Autodesk Inventor part; units mm, degrees
ref_plane "YZ Plane" through (0, 0, 0) normal (1, 0, 0) x (0, 1, 0)
ref_plane "XZ Plane" through (0, 0, 0) normal (0, 1, 0) x (-1, 0, 0)
ref_plane "XY Plane" through (0, 0, 0) normal (0, 0, 1) x (1, 0, 0)
sketch "Sketch2" plane through (0, 0, 0) normal (1, 0, 0) x (0, 1, 0)
  line L0 (0, 0) -> (30, 0)
  line L1 (30, 60) -> (30, -60)
  line L2 (30, 60) -> (27, 60)
  line L3 (27, 60) -> (27, -60)
  line L4 (27, -60) -> (30, -60)
  line L5 (27, 60) -> (0, 60)
  line L6 (0, 60) -> (5, 60)
  line L7 (5, 60) -> (5, 54)
  line L8 (5, 54) -> (27, 54)
  line L9 (27, -60) -> (0, -60)
  line L10 (0, -60) -> (5, -60)
  line L11 (5, -60) -> (5, -54)
  line L12 (5, -54) -> (27, -54)
  line L13 (0, 60) -> (0, -60)
  line L14 (27, 0) -> (28, 0)
  line L15 (28, 0) -> (28, -3)
  line L16 (28, -3) -> (27, -3)
  line L17 (28, 0) -> (28, 2)
  line L18 (28, 2) -> (30, 2)
  line L19 (30, 2) -> (28, 0)
  line L20 (28, 0) -> (28, -2)
  line L21 (28, -2) -> (30, -2)
  line L22 (30, -2) -> (28, 0)
  line L23 (5, -54) -> (0, -54)
  dimension "d12" = 30
  dimension "d13" = 120
  dimension "d14" = 3
  dimension "d15" = 5
  dimension "d16" = 6
  dimension "d17" = 6
  dimension "d26" = 1
  dimension "d27" = 3
  dimension "d28" = 2
  dimension "d29" = 2
revolve "Revolution1" add sketch "Sketch2" angle 360 about axis through (0, 0, 60) along (0, 0, -1) contours L23 L11 L9 L13 | L22 L21 L15 | L16 L15 L21 L1 L4 L3 | L12 L3 L9 L11
fillet "Fillet2" radius 3 1 edges at (0, -30, -60)
fillet "Fillet3" radius 3 1 edges at (0, -27, -54)
properties part number "Plenum"
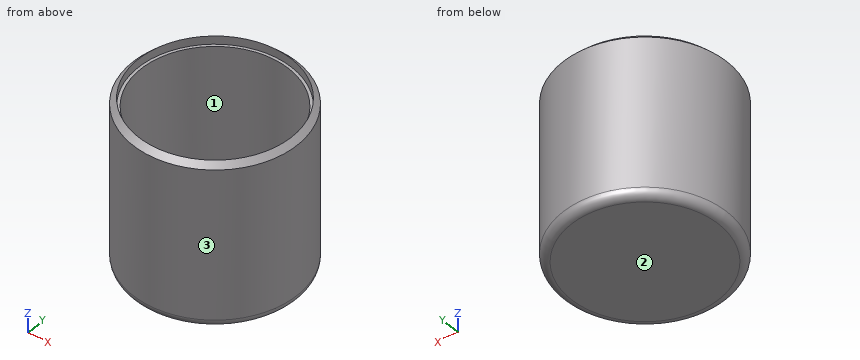
Build history of the part. All positions in model axes, mm. Face numbers are marked on the shaded views. Give positions to 0.01 mm unless a question says otherwise; leave off trailing zeros. Loops run counter-clockwise (first coordinate to the right, second up) from the corner with the lowest first, then second, coordinate; pieces in that order, holes last.
Item 1: Drill centre lines: line 1 (X direction, y = 0, z = -2); line 2 (X direction, y = 0, z = -23); line 3 (Z direction, x = 14, y = -6). Where is each one in solid material? Low to high.
Answers follow:
line 1: x = -30 to -28, 28 to 30
line 2: x = -30 to -27, 27 to 30
line 3: z = -60 to -54
Item 2: Pull direction X, two halves, no side cores. Call the marked faces 1, 2 and 3: released by +X, released by -X, zero draft, split by the parting line, or undercut.
Answers follow:
face 1: undercut
face 2: zero draft
face 3: split by the parting line
Item 3: Slice it at A-A, the plane y = 0. List the corners of the cut face in (x, z), and give its area (3 significant figures).
Answers follow:
outline: (-30, -57) arc R3 ccw to (-27, -60) - (27, -60) arc R3 ccw to (30, -57) - (30, -2) - (28, 0) - (28, -3) - (27, -3) - (27, -51) arc R3 cw to (24, -54) - (-24, -54) arc R3 cw to (-27, -51) - (-27, -3) - (-28, -3) - (-28, 0) - (-30, -2) - close
area: 674 mm2
Item 4: Flat gauge pins, fed straight in: pin 1 (8 mm diameter, centred on y = 10, z = -31, fed in from +X); pin 2 (8 mm diameter, centred on y = -3.5, z = -11, fed in from -X); pin 3 (1.5 mm diameter, centred on y = -12, z = -16, fed in from +X). Where does each tip first touch, or does it go through?
Answers follow:
pin 1: stops at x = 29.39
pin 2: stops at x = -30
pin 3: stops at x = 27.81
